from build123d import *

# Parameters (mm, degrees)
BOSS_EXTRUDE1_DEPTH  = 3
SKETCH2_R            = 1.575
CUT_EXTRUDE1_DEPTH   = 4
SKETCH3_R            = 1.75
CUT_EXTRUDE2_DEPTH   = 4
LPATTERN1_COUNT      = 2
LPATTERN1_PITCH      = 70
LPATTERN1_COUNT_DIR2 = 2
LPATTERN1_PITCH_DIR2 = 90
SKETCH4_R            = 1.5
CUT_EXTRUDE3_DEPTH   = 4
SKETCH5_W            = 30
SKETCH5_H            = 45
CUT_EXTRUDE4_DEPTH   = 4


with BuildPart() as part:
    # Sketch1 → Boss-Extrude1 (new body)
    with BuildSketch(Plane(origin=(0, 0, 0), x_dir=(1, 0, 0), z_dir=(0, 1, 0))):
        with BuildLine():
            Line((-45, 40), (45, 40))
            ThreePointArc((45, 40), (48.535533906, 38.535533906), (50, 35))
            Line((50, 35), (50, -35))
            ThreePointArc((50, -35), (48.535533906, -38.535533906), (45, -40))
            Line((45, -40), (-45, -40))
            ThreePointArc((-45, -40), (-48.535533906, -38.535533906), (-50, -35))
            Line((-50, -35), (-50, 35))
            ThreePointArc((-50, 35), (-48.535533906, 38.535533906), (-45, 40))
        make_face()
    extrude(amount=BOSS_EXTRUDE1_DEPTH)

    # Sketch2 → Cut-Extrude1 (cut)
    with BuildSketch(Plane(origin=(0, 3, 0), x_dir=(1, 0, 0), z_dir=(0, 1, 0))):
        with Locations((-36.5, 9)):
            Circle(SKETCH2_R)
        with Locations((-36.5, -9)):
            Circle(SKETCH2_R)
        with Locations((36.5, -9)):
            Circle(SKETCH2_R)
        with Locations((36.5, 9)):
            Circle(SKETCH2_R)
    extrude(amount=-CUT_EXTRUDE1_DEPTH, mode=Mode.SUBTRACT)

    # Sketch3 → Cut-Extrude2 (cut, through all)
    with BuildSketch(Plane(origin=(0, 3, 0), x_dir=(1, 0, 0), z_dir=(0, 1, 0))):
        with Locations((-45, -35)):
            Circle(SKETCH3_R)
    cut_extrude2 = extrude(amount=-CUT_EXTRUDE2_DEPTH, mode=Mode.SUBTRACT)

    # LPattern1: Cut-Extrude2 2 × 2
    with Locations(*[(j * LPATTERN1_PITCH_DIR2, 0, -i * LPATTERN1_PITCH) for i in range(LPATTERN1_COUNT) for j in range(LPATTERN1_COUNT_DIR2) if (i, j) != (0, 0)]):
        add(cut_extrude2, mode=Mode.SUBTRACT)

    # Sketch4 → Cut-Extrude3 (cut, through all)
    with BuildSketch(Plane(origin=(0, 3, 0), x_dir=(1, 0, 0), z_dir=(0, 1, 0))):
        with Locations((-39.4, 28)):
            Circle(SKETCH4_R)
        with Locations((39.4, 28)):
            Circle(SKETCH4_R)
        with Locations((39.4, -28)):
            Circle(SKETCH4_R)
        with Locations((-39.4, -28)):
            Circle(SKETCH4_R)
    extrude(amount=-CUT_EXTRUDE3_DEPTH, mode=Mode.SUBTRACT)

    # Sketch5 → Cut-Extrude4 (cut, through all)
    with BuildSketch(Plane(origin=(0, 3, 0), x_dir=(1, 0, 0), z_dir=(0, 1, 0))):
        Rectangle(SKETCH5_W, SKETCH5_H)
    extrude(amount=-CUT_EXTRUDE4_DEPTH, mode=Mode.SUBTRACT)


solid = part.part
The model under review builds one solid part; all positions refer to its coordinate system, in mm. A direction names the side the tool comes from. Give positions to 0.01 mm unless a question says otherwise; leave off trailing zeros. Write each loop counter-clockwise with the first axis right and the second up, starting at its lowest first coordinate (ties: lowest second). Pieces come first, ordered by that corner, then holes. Notation, with made-up numbers: M -9.5,16 L 44.5,16 A14 cw 44.5,33 Z; hole C -17.5,50 d3. An arc over 180 degrees is marked long. One line per question, with ' | ' between items. Start each with the question number.
Item 1: We need section D-D on y = 0.6. Give the number of separate pieces and of enclosed holes in the cut face, plus the area to 3 significant figures.
Item 2: For pin 1 (3 mm diameter, centred on x = 36.5, z = 9, fed in from -Y) (3 decimals); pin 2 (3.5 mm diameter, centred on x = -36.5, z = 9, fed in from -Y), all flat-tipped, find the tip position at first contact; note any pin that passes through.
Item 3: We need section B-B on x = 4. Write out the cut boundary in (y, z).
Item 4: Wall thickness on line 1 (X direction, y = 2, z = 9) (3 decimals); line 2 (Z direction, x = -39.4, y = 1.4); line 3 (Z direction, x = 36.5, y = 1) (3 decimals): over which ranges is each line inside the solid? List them lowest first. Write a range as from..to.
Item 5: Draft analysis for pull direction Z (two halves, no side actions). For faces 1 (the cylindrical face through (49, 1, 38)), 2 (the flat face through (50, 1, 0)), 3 (the cylindrical face through (-40.51, 1.52, -29.01)), state which applies: released by +Z, released by -Z, zero draft, split by the parting line, or undercut.
Item 6: We need section A-A on x = 39.4. Write out the cut boundary in (y, z).
Item 7: For faces 4 (the flat face through (-15, 2, 0)), 5 (the flat face through (1, 1, 40)), list the 3-axis set-ups (+Z, -Z, +X, -X, +Y, -Y) from which the entire face can be reached by the end or side of a thin tool; tool diameter is ignored.
Item 8: We need section C-C on z = 20. Write out the cut boundary in (x, y), plus the area to 3 significant figures.
Results found:
1) separate pieces: 1 | enclosed holes: 13 | area: 6,530 mm2
2) pin 1: passes through | pin 2: stops at y = 0
3) outline: M 0,-40 L 3,-40 L 3,-22.5 L 0,-22.5 Z; M 0,22.5 L 3,22.5 L 3,40 L 0,40 Z
4) line 1: x = -50..-38.075, -34.925..-15, 15..34.925, 38.075..50 | line 2: z = -40..-29.5, -26.5..26.5, 29.5..40 | line 3: z = -40..-10.575, -7.425..7.425, 10.575..40
5) face 1: released by +Z | face 2: zero draft | face 3: undercut
6) outline: M 0,-40 L 3,-40 L 3,-29.5 L 0,-29.5 Z; M 0,-26.5 L 3,-26.5 L 3,26.5 L 0,26.5 Z; M 0,29.5 L 3,29.5 L 3,40 L 0,40 Z
7) face 4: +Y, -Y | face 5: +Z, +X, -X, +Y, -Y
8) outline: M -50,0 L -15,0 L -15,3 L -50,3 Z; M 15,0 L 50,0 L 50,3 L 15,3 Z | area: 210 mm2
